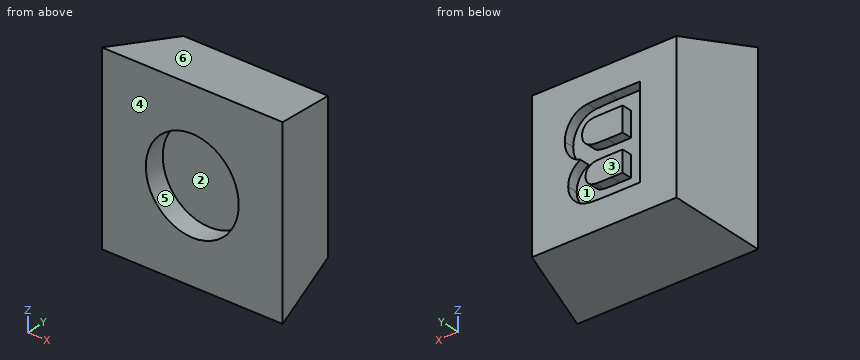
```python
from build123d import *

# Parameters (mm, degrees)
SKETCH1_W           = 7
SKETCH1_H           = 7
BOSS_EXTRUDE1_DEPTH = 3
CUT_EXTRUDE1_DEPTH  = 7
CUT_EXTRUDE2_DEPTH  = 11
SKETCH4_R           = 1.8
CUT_EXTRUDE3_DEPTH  = 0.8
CUT_EXTRUDE4_DEPTH  = 0.4


with BuildPart() as part:
    # Sketch1 → Boss-Extrude1 (new body)
    with BuildSketch(Plane(origin=(0, 0, 0), x_dir=(1, 0, 0), z_dir=(0, 1, 0))):
        with Locations((3.5, 3.5)):
            Rectangle(SKETCH1_W, SKETCH1_H)
    extrude(amount=BOSS_EXTRUDE1_DEPTH)

    # Sketch2 → Cut-Extrude1 (cut)
    with BuildSketch(Plane.XY):
        Polygon((0, 0), (0.7, 3), (0, 3), align=None)
        Polygon((7, 0), (6.3, 3), (7, 3), align=None)
    extrude(amount=-CUT_EXTRUDE1_DEPTH, mode=Mode.SUBTRACT)

    # Sketch3 → Cut-Extrude2 (cut)
    with BuildSketch(Plane(origin=(0, 0, 0), x_dir=(0, 0, -1), z_dir=(1, 0, 0))):
        Polygon((0, 0), (0.7, 3), (0, 3), align=None)
        Polygon((7, 3), (6.3, 3), (7, 0), align=None)
    extrude(amount=CUT_EXTRUDE2_DEPTH, mode=Mode.SUBTRACT)

    # Sketch4 → Cut-Extrude3 (cut)
    with BuildSketch(Plane.XZ):
        with Locations(Location((3.5, -3.5, 0), (0, 0, 270))):
            Circle(SKETCH4_R)
    extrude(amount=-CUT_EXTRUDE3_DEPTH, mode=Mode.SUBTRACT)

    # Sketch5 → Cut-Extrude4 (cut)
    with BuildSketch(Plane(origin=(0, 3, 0), x_dir=(1, 0, 0), z_dir=(0, 1, 0))):
        with BuildLine():
            Line((2.111509743, 5.252535384), (3.521465672, 5.252535384))
            add(Edge.make_bspline(
                [(3.521465672, 5.252535384), (3.555352929, 5.252333756), (3.620793103, 5.251944389), (3.715699078, 5.250859268), (3.803790562, 5.247672529), (3.88520473, 5.244936095), (3.959670809, 5.238536714), (4.027774054, 5.233508957), (4.089300044, 5.226592072), (4.161779262, 5.215398498), (4.246059792, 5.197987684), (4.341252586, 5.165782389), (4.43148602, 5.125545022), (4.515403802, 5.074389368), (4.593284686, 5.014559615), (4.665724305, 4.946532312), (4.729381186, 4.867558536), (4.786703202, 4.781364769), (4.835087081, 4.687878618), (4.868405373, 4.587306133), (4.88966817, 4.481491325), (4.892245345, 4.408956406), (4.893561025, 4.37192641)],
                knots=[0, 0, 0, 0, 1.096610875, 2.117681168, 3.071055591, 3.949137991, 4.753059115, 5.489127199, 6.15892391, 6.75575099, 7.862330316, 8.938514814, 10.001276227, 11.05313779, 12.110449801, 13.174958802, 14.260456508, 15.384725817, 16.521138801, 17.654729897, 18.802709851, 20, 20, 20, 20], degree=3))
            add(Edge.make_bspline(
                [(4.893561025, 4.37192641), (4.892196479, 4.331601681), (4.889505896, 4.252090262), (4.864462524, 4.135494667), (4.824571342, 4.023939737), (4.768250724, 3.919235161), (4.699269413, 3.823150089), (4.617676049, 3.738775738), (4.524669493, 3.666625119), (4.454832509, 3.630722743), (4.419602692, 3.612611506)],
                knots=[0, 0, 0, 0, 1.023065178, 2.01725758, 3.014298905, 4.023406433, 5.026736079, 6.009055718, 6.99565244, 8, 8, 8, 8], degree=3))
            add(Edge.make_bspline(
                [(4.419602692, 3.612611506), (4.443330648, 3.604529528), (4.490246921, 3.588549379), (4.557400348, 3.559205258), (4.620319472, 3.52517498), (4.678972699, 3.487531632), (4.733805186, 3.446000029), (4.783214944, 3.399203081), (4.83003713, 3.349803196), (4.871143379, 3.295320645), (4.908350842, 3.238361247), (4.939934418, 3.17803347), (4.967283165, 3.115788352), (4.990155428, 3.050995933), (5.006459358, 2.983221651), (5.019523083, 2.913319286), (5.02620612, 2.840804369), (5.027514255, 2.791842338), (5.02817641, 2.767058621)],
                knots=[0, 0, 0, 0, 1.072651974, 2.1209089, 3.132484228, 4.131466326, 5.101889999, 6.071643115, 7.041396231, 8.011819904, 8.988565287, 9.95070344, 10.922775742, 11.897213062, 12.887138018, 13.903598663, 14.938838629, 16, 16, 16, 16], degree=3))
            add(Edge.make_bspline(
                [(5.02817641, 2.767058621), (5.026768086, 2.727480727), (5.02395794, 2.64850764), (5.002958076, 2.530696633), (4.96749134, 2.414960489), (4.919462058, 2.302050025), (4.859804392, 2.195584607), (4.789667704, 2.098381872), (4.707836651, 2.01380613), (4.617215838, 1.939282584), (4.515099833, 1.877587714), (4.401575881, 1.830197397), (4.277361379, 1.794394944), (4.18985285, 1.782501682), (4.144762948, 1.776373525)],
                knots=[0, 0, 0, 0, 0.975059807, 1.945618526, 2.93861228, 3.952760547, 4.963632603, 5.940527786, 6.897802811, 7.855787948, 8.824773195, 9.82606706, 10.879852914, 12, 12, 12, 12], degree=3))
            add(Edge.make_bspline(
                [(4.144762948, 1.776373525), (4.127472996, 1.774915024), (4.087782581, 1.771566924), (4.020469845, 1.767404325), (3.937705498, 1.764257864), (3.839561406, 1.760537572), (3.725735437, 1.757851413), (3.596486285, 1.756017129), (3.451593418, 1.75363659), (3.349925557, 1.752915159), (3.296405576, 1.752535384)],
                knots=[0, 0, 0, 0, 0.490565993, 1.126131979, 1.906526787, 2.832178623, 3.902933831, 5.125497984, 6.486805064, 8, 8, 8, 8], degree=3))
            Line((3.296405576, 1.752535384), (2.111509743, 1.752535384))
            Line((2.111509743, 1.752535384), (2.111509743, 5.252535384))
        make_face()
        with BuildLine():
            Line((2.784586666, 4.669202051), (2.784586666, 3.861509743))
            Line((2.784586666, 3.861509743), (3.271866313, 3.861509743))
            add(Edge.make_bspline(
                [(3.271866313, 3.861509743), (3.306221586, 3.861434055), (3.371661079, 3.861289884), (3.464674551, 3.862255994), (3.547646114, 3.862707017), (3.620337221, 3.8640307), (3.682732948, 3.866215267), (3.734608475, 3.868396735), (3.776263571, 3.870048358), (3.800518366, 3.872406802), (3.811028974, 3.873428813)],
                knots=[0, 0, 0, 0, 1.528479216, 2.911428072, 4.138414629, 5.21998762, 6.145918986, 6.915989543, 7.530253335, 8, 8, 8, 8], degree=3))
            add(Edge.make_bspline(
                [(3.811028974, 3.873428813), (3.841339923, 3.877989922), (3.899595708, 3.886756091), (3.981115359, 3.912443032), (4.051822858, 3.949594446), (4.112503082, 3.995838149), (4.16067052, 4.052573755), (4.196017974, 4.117840239), (4.216698833, 4.191911851), (4.219190867, 4.243956456), (4.220484102, 4.270964871)],
                knots=[0, 0, 0, 0, 1.162079002, 2.233444551, 3.225172046, 4.179556897, 5.110707885, 6.027301426, 6.976273101, 8, 8, 8, 8], degree=3))
            add(Edge.make_bspline(
                [(4.220484102, 4.270964871), (4.219672292, 4.297045189), (4.21811382, 4.347112917), (4.198753979, 4.418001877), (4.169647913, 4.481665844), (4.127102602, 4.536540746), (4.073714805, 4.582883197), (4.008370927, 4.619083019), (3.931384749, 4.643991925), (3.875931131, 4.652704095), (3.846786185, 4.65728298)],
                knots=[0, 0, 0, 0, 1.044241546, 2.004684189, 2.928111627, 3.838334562, 4.769594837, 5.748424953, 6.81663206, 8, 8, 8, 8], degree=3))
            add(Edge.make_bspline(
                [(3.846786185, 4.65728298), (3.835340353, 4.658308087), (3.808280354, 4.660731624), (3.761249742, 4.662307099), (3.701429573, 4.664524478), (3.628514928, 4.666688526), (3.542503834, 4.668009799), (3.443640912, 4.668455112), (3.331930575, 4.669425441), (3.253169995, 4.669279261), (3.211569839, 4.669202051)],
                knots=[0, 0, 0, 0, 0.433943041, 1.02591908, 1.776648879, 2.694999143, 3.780816848, 5.02540149, 6.428861738, 8, 8, 8, 8], degree=3))
            Line((3.211569839, 4.669202051), (2.784586666, 4.669202051))
        make_face(mode=Mode.SUBTRACT)
        with BuildLine():
            Line((2.784586666, 3.27817641), (2.784586666, 2.335868717))
            Line((2.784586666, 2.335868717), (3.471686025, 2.335868717))
            add(Edge.make_bspline(
                [(3.471686025, 2.335868717), (3.503705507, 2.335709884), (3.564476207, 2.33540843), (3.651169443, 2.337427531), (3.728560529, 2.338093302), (3.79701169, 2.341414873), (3.856163227, 2.343927607), (3.906258531, 2.347060152), (3.946906458, 2.352041803), (3.970893783, 2.355909309), (3.98140157, 2.357603493)],
                knots=[0, 0, 0, 0, 1.504773752, 2.85595359, 4.075347731, 5.141676974, 6.076328919, 6.858106537, 7.499786952, 8, 8, 8, 8], degree=3))
            add(Edge.make_bspline(
                [(3.98140157, 2.357603493), (4.008085962, 2.36323372), (4.059931656, 2.374172812), (4.13178912, 2.405562615), (4.196552287, 2.445370583), (4.252642198, 2.496532162), (4.298745197, 2.557822327), (4.332034841, 2.629376077), (4.352110737, 2.710351547), (4.354073968, 2.767404519), (4.355099486, 2.797206858)],
                knots=[0, 0, 0, 0, 1.031056579, 2.003262591, 2.954260215, 3.900917722, 4.862741126, 5.841340256, 6.872396835, 8, 8, 8, 8], degree=3))
            add(Edge.make_bspline(
                [(4.355099486, 2.797206858), (4.354271867, 2.82276493), (4.352661002, 2.872510733), (4.336892789, 2.943762046), (4.311385128, 3.008909067), (4.275862523, 3.067507228), (4.231481376, 3.120292471), (4.17661735, 3.164466336), (4.113275558, 3.201270071), (4.052892173, 3.225515958), (3.995633073, 3.241071138), (3.941019912, 3.251275641), (3.875199891, 3.25935328), (3.798492104, 3.266186067), (3.710585277, 3.271650146), (3.611715662, 3.275957666), (3.501607357, 3.277760533), (3.424477404, 3.278033382), (3.384045801, 3.27817641)],
                knots=[0, 0, 0, 0, 0.992165387, 1.931134082, 2.820086661, 3.700270762, 4.583075858, 5.486803518, 6.423132184, 7.421722103, 8.005700193, 8.727213115, 9.57900282, 10.582332745, 11.720121093, 13.002085041, 14.428489784, 16, 16, 16, 16], degree=3))
            Line((3.384045801, 3.27817641), (2.784586666, 3.27817641))
        make_face(mode=Mode.SUBTRACT)
    extrude(amount=-CUT_EXTRUDE4_DEPTH, mode=Mode.SUBTRACT)


solid = part.part
```
Part model, mm, in its own coordinate system. Face numbers are marked on the shaded views. A direction names the side the tool comes from. Round coordinates to 2 decimals unless told otherwise and drop trailing zeros. Loops run counter-clockwise (first coordinate to the right, second up) from the corner with the lowest first, then second, coordinate; pieces in that order, holes last. Notation, with made-up numbers: (75, 18.25) -> (128, 18.25) arc R18 cw to (128, 42.25) -> close; hole circle Ø5 at (33, 6). An arc over 180 degrees is marked (long way). Use CSV: the item, a comma, the result in double quotes. Start each with the question number.
1) Which spindle directions (+Z, -Z, +X, -X, +Y, -Y) get a long thin tool onto all of the face, cutting with end or side? Do the marked faces 1, 2 and 3. Say none if no direction does.
2) Wall check: L1, parallel to Z at x = 3.5, y = 2.9; L2, parallel to Z at x = 4.75, y = 2.85 (3 decimals); L3, parallel to Y at x = 2.5, z = -3.5. Give the ranges that are in metal, low to high. Write a range as [from, to].
3) Cut at A-A, the plane z = -5.75. Write the cut outline in (x, y).
4) Drop a flat-ended pin along its axis: P1, Ø1, axis at y = 1.5, z = -4.5, coming from the +X side. Give the stop position or say it passes through.
5) Cut at B-B, the plane x = 1. Write the cut outline in (y, z).
6) Pull direction Z, two halves, no side cores. Call the marked faces 4, 5 and 6: +Z half, -Z half, draft (parallel to the pull), parting line (faces both ways), or undercut.
Determined:
1,face 1,"+Y"
1,face 2,"-Y"
1,face 3,"+Z, -Z, +X, -X, +Y"
2,L1,"z = [-6.32, -5.25], [-4.67, -3.86], [-3.28, -2.34], [-1.75, -0.68]"
2,L2,"z = [-6.335, -4.836], [-3.896, -3.43], [-2.058, -0.665]"
2,L3,"y = [0.8, 2.6]"
3,outline,"(0, 0) -> (7, 0) -> (6.3, 3) -> (0.7, 3) -> close"
4,P1,"stops at x = 6.77"
5,outline,"(0, -7) -> (3, -6.3) -> (3, -0.7) -> (0, 0) -> close"
6,face 4,"draft"
6,face 5,"undercut"
6,face 6,"+Z half"
